```python
from build123d import *

# Parameters (mm, degrees)
SKETCH_1_R      = 2.4
SKETCH_1_R_2    = 3.8
EXTRUDE_1_DEPTH = 4
SKETCH_1_3_R    = 3.8
SKETCH_1_3_R_2  = 1.4
EXTRUDE_2_DEPTH = 8


with BuildPart() as part:
    # Sketch 1 → Extrude 1 (new body)
    with BuildSketch(Plane.XY):
        with BuildLine():
            Line((-7.5, 15), (7.5, 15))
            ThreePointArc((7.5, 15), (22.5, 0), (7.5, -15))
            Line((7.5, -15), (-7.5, -15))
            ThreePointArc((-7.5, -15), (-22.5, 0), (-7.5, 15))
        make_face()
        with Locations((-10, 0)):
            Circle(SKETCH_1_R, mode=Mode.SUBTRACT)
        with Locations((10, 0)):
            Circle(SKETCH_1_R, mode=Mode.SUBTRACT)
        with Locations((0, 5)):
            Circle(SKETCH_1_R_2, mode=Mode.SUBTRACT)
    extrude(amount=EXTRUDE_1_DEPTH)

    # Sketch 1_3 → Extrude 2 (add)
    with BuildSketch(Plane.XY):
        with Locations((0, 5)):
            Circle(SKETCH_1_3_R)
        with Locations((0, 5)):
            Circle(SKETCH_1_3_R_2, mode=Mode.SUBTRACT)
    extrude(amount=EXTRUDE_2_DEPTH)


solid = part.part
```
Geometry: final body of the model. Coordinates: model frame, mm. Coordinates: 2 decimals unless noted, no trailing zeros. Order: outer loops, then holes, each group sorted by start corner. A loop starts at its lowest first (then second) coordinate and runs counter-clockwise, first axis right, second up. Notation, with made-up numbers: (69.5, 56) - (109.5, 56) arc R34 cw to (109.5, 86) - close; hole circle Ø4 at (-10, 33.25). An arc over 180 degrees is marked (long way). Return JSON: item names as keys, results as strings. Group by question number.
1. Material intervals for line 1 along X through (y, z) = (-1.5, 2.25); line 2 along Z through (x, y) = (8, 10); line 3 along Y through (x, z) = (10, 2.65), sorted ascending. Write a range as [from, to].
2. Cut plane A-A (x = 0). Output: boundary loops of the cut face in (y, z), plus the area to 3 significant figures.
3. Pull-direction query (Y, two-part tool) for faces 1 (the face through (-1.03, 5.95, 3.94)), 2 (the face through (0, 0, 4)), 3 (the face through (3.625, 6.141, 5.972)); classes: pulls with the +Y half, pulls with the -Y half, needs draft (parallel to the pull), parting line crosses it, or undercut.
4. Cut plane B-B (y = 5). Output: boundary loops of the cut face in (x, z).
5. Cut plane D-D (x = 10). Output: boundary loops of the cut face in (y, z).
6. Pin query (flat end, axial travel): pin 1 (3 mm diameter, centred on x = 10, y = 1.5, fed in from +Z); pin 2 (4 mm diameter, centred on x = -10.5, z = 3, fed in from -Y); pin 3 (3 mm diameter, centred on x = -10, y = 0, fed in from +Z). Return the tip coordinate at first contact, or that it passes through.
7. Cut plane C-C (z = 4.5). Output: boundary loops of the cut face in (x, y).
Resolved:
{
 "1": {"line 1": "x = [-22.42, -11.87], [-8.13, 8.13], [11.87, 22.42]", "line 2": "z = [0, 4]", "line 3": "y = [-14.79, -2.4], [2.4, 14.79]"},
 "2": {"outline": "(-15, 0) - (3.6, 0) - (3.6, 8) - (1.2, 8) - (1.2, 4) - (-15, 4) - close; (6.4, 0) - (15, 0) - (15, 4) - (8.8, 4) - (8.8, 8) - (6.4, 8) - close", "area": "128 mm²"},
 "3": {"face 1": "undercut", "face 2": "needs draft", "face 3": "parting line crosses it"},
 "4": {"outline": "(-21.64, 0) - (-1.4, 0) - (-1.4, 8) - (-3.8, 8) - (-3.8, 4) - (-21.64, 4) - close; (1.4, 0) - (21.64, 0) - (21.64, 4) - (3.8, 4) - (3.8, 8) - (1.4, 8) - close"},
 "5": {"outline": "(-14.79, 0) - (-2.4, 0) - (-2.4, 4) - (-14.79, 4) - close; (2.4, 0) - (14.79, 0) - (14.79, 4) - (2.4, 4) - close"},
 "6": {"pin 1": "stops at z = 4", "pin 2": "stops at y = -14.97", "pin 3": "passes through"},
 "7": {"outline": "circle Ø7.6 at (0, 5); hole circle Ø2.8 at (0, 5)"}
}
